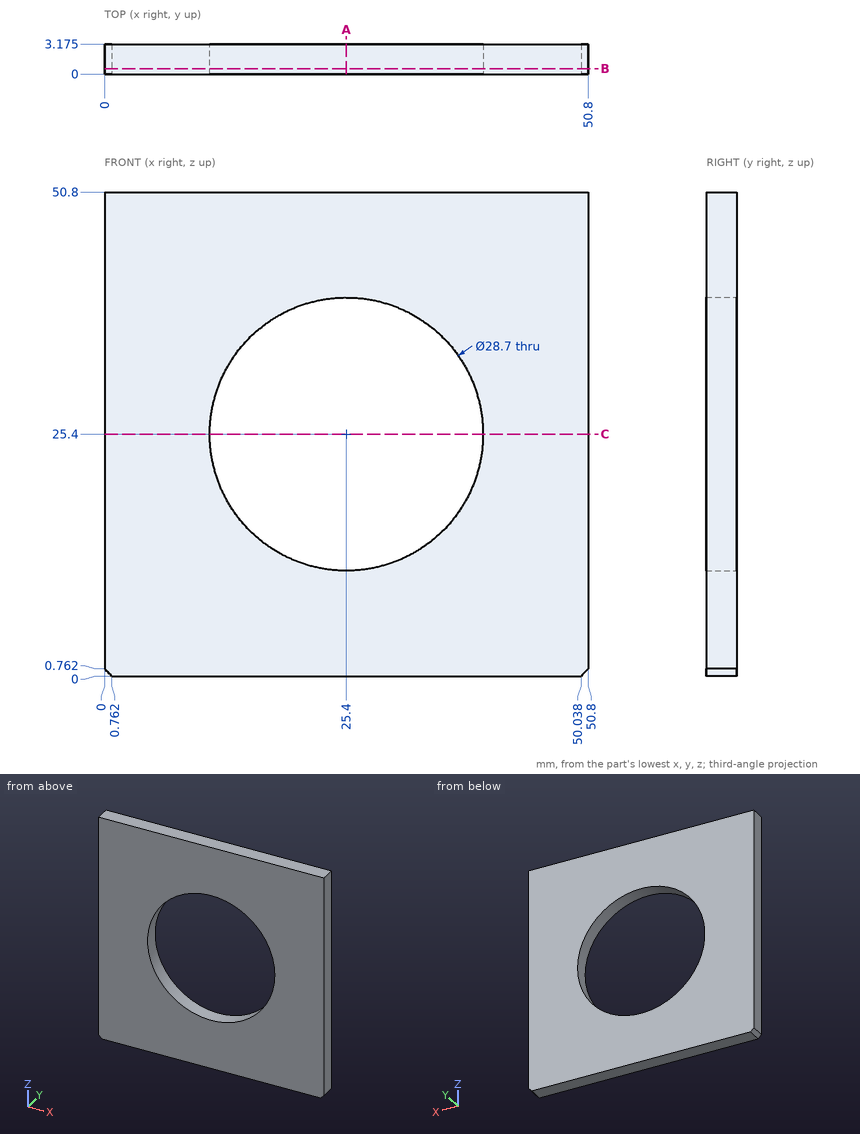
Geometry: see drawing. Coordinates: mm, zero at the bounding-box minimum. Coordinates: 2 decimals unless noted, no trailing zeros. Order: outer loops, then holes, each group sorted by start corner. A loop starts at its lowest first (then second) coordinate and runs counter-clockwise, first axis right, second up. Notation, with made-up numbers: M 48,9.5 L 74,9.5 A15 cw 74,27.5 Z; hole C 36.25,-2 d5. An arc over 180 degrees is marked long. Answer in a Markdown table with one row per item. Add a question column.
Q1. Section query C-C on z = 25.4. Return the cut outline in (x, y) (3 decimals), and give its area (3 significant figures).
Q2. Section query B-B on y = 0.6. Return the cut outline in (x, z), and give its area (3 significant figures).
Q3. Section query A-A on x = 25.4. Return the cut outline in (y, z) (3 decimals).
Q4. Line query: L1, parallel to Z at x = 25.4, y = 1.8; L2, parallel to X at y = 2.7, z = 19.5. Output: solid intervals per line, ascending.
Completed:
| question | item | result |
|---|---|---|
| 1 | outline | M 0,0 L 11.05,0 L 11.05,3.175 L 0,3.175 Z; M 39.75,0 L 50.8,0 L 50.8,3.175 L 39.75,3.175 Z |
| 1 | area | 70.2 mm2 |
| 2 | outline | M 0,0.76 L 0.76,0 L 50.04,0 L 50.8,0.76 L 50.8,50.8 L 0,50.8 Z; hole C 25.4,25.4 d28.7 |
| 2 | area | 1,930 mm2 |
| 3 | outline | M 0,0 L 3.175,0 L 3.175,11.05 L 0,11.05 Z; M 0,39.75 L 3.175,39.75 L 3.175,50.8 L 0,50.8 Z |
| 4 | L1 | z = 0 to 11.05, 39.75 to 50.8 |
| 4 | L2 | x = 0 to 12.32, 38.48 to 50.8 |
